Work out the finished part from the listing and answer in its coordinate system (mm). A direction names the side the tool comes from. Give positions to 0.01 mm unless a question says otherwise; leave off trailing zeros. Loops run counter-clockwise (first coordinate to the right, second up) from the corner with the lowest first, then second, coordinate; pieces in that order, holes last. Notation, with made-up numbers: M -9,84 L 7,84 A20 ccw 7,91 Z; hole C 23,85.5 d4. An arc over 180 degrees is marked long. Answer as a JSON object with one key per item and string values. Group by question number.
```python
from build123d import *

# Parameters (mm, degrees)
SKETCH_1_R          = 14
SKETCH_1_R_2        = 1.5
EXTRUDE_1_DEPTH     = 3
SKETCH_2_R          = 5.5
CUT_EXTRUDE_1_DEPTH = 11
CUT_EXTRUDE_2_DEPTH = 11
SKETCH_6_R          = 1.5
CUT_EXTRUDE_3_DEPTH = 11
SKETCH_4_R          = 1.5
EXTRUDE_2_DEPTH     = 3
FILLET_1_R          = 3


with BuildPart() as part:
    # 草图1 → 凸台-拉伸1 (new body)
    # profile 1 of 2: a face of its own
    with BuildSketch(Plane.XY):
        with BuildLine():
            Line((-14, 27.287521581), (-14, 0))
            ThreePointArc((-14, 0), (0, 14), (14, 0))
            Line((14, 0), (14, 27.287521581))
            Line((14, 27.287521581), (-14, 27.287521581))
        make_face()
    # profile 2 of 2: a face of its own
    with BuildSketch(Plane.XY):
        Circle(SKETCH_1_R)
        with Locations((0, -8)):
            Circle(SKETCH_1_R_2, mode=Mode.SUBTRACT)
        with Locations((8, 0)):
            Circle(SKETCH_1_R_2, mode=Mode.SUBTRACT)
        with Locations((-8, 0)):
            Circle(SKETCH_1_R_2, mode=Mode.SUBTRACT)
    extrude(amount=EXTRUDE_1_DEPTH)

    # 草图2 → 切除-拉伸1 (cut)
    with BuildSketch(Plane.XY.offset(3)):
        Circle(SKETCH_2_R)
    extrude(amount=-CUT_EXTRUDE_1_DEPTH, mode=Mode.SUBTRACT)

    # 草图3 → 切除-拉伸2 (cut)
    with BuildSketch(Plane.XY.offset(3)):
        Polygon((14, 27.287521581), (22.040424941, 27.287521581), (22.040424941, 21.507521581), (-23.523215241, 21.507521581), (-23.523215241, 27.287521581), align=None)
    extrude(amount=-CUT_EXTRUDE_2_DEPTH, mode=Mode.SUBTRACT)

    # 草图6 → 切除-拉伸3 (cut)
    with BuildSketch(Plane.XY.offset(3)):
        with Locations((10, 14.007521581)):
            Circle(SKETCH_6_R)
        with Locations((-10, 14.007521581)):
            Circle(SKETCH_6_R)
    extrude(amount=-CUT_EXTRUDE_3_DEPTH, mode=Mode.SUBTRACT)

    # 草图4 → 凸台-拉伸2 (add)
    with BuildSketch(Plane.XY.offset(3)):
        Polygon((14, 21.507521581), (34.450975214, 21.507521581), (34.450975214, 6.507521581), (14, 6.507521581), (-14, 6.507521581), (-34.450975214, 6.507521581), (-34.450975214, 21.507521581), (-14, 21.507521581), align=None)
        with Locations((10, 14.007521581)):
            Circle(SKETCH_4_R, mode=Mode.SUBTRACT)
        with Locations((28, 14.007521581)):
            Circle(SKETCH_4_R, mode=Mode.SUBTRACT)
        with Locations((-10, 14.007521581)):
            Circle(SKETCH_4_R, mode=Mode.SUBTRACT)
        with Locations(Location((-28, 14.007521581, 0), (0, 0, 180))):
            Circle(SKETCH_4_R, mode=Mode.SUBTRACT)
    extrude(amount=-EXTRUDE_2_DEPTH)

    # 圆角1
    fillet_1_edges = [part.edges().sort_by_distance(p)[0] for p in [
        (-34.450975214, 21.507521581, 1.5),
        (-14, 6.507521581, 1.5),
        (34.450975214, 21.507521581, 1.5),
        (14, 6.507521581, 1.5),
        (34.450975214, 6.507521581, 1.5),
        (-34.450975214, 6.507521581, 1.5),
    ]]
    fillet(fillet_1_edges, radius=FILLET_1_R)


solid = part.part
```
Item 1: Find the intervals of material crossed by probe 1 along X at (y, z) = (14, 0.95); probe 2 along Y at (x, z) = (28, 2.3); probe 3 along Y at (x, z) = (8, 1), in increasing order. Write a range as [from, to].
Item 2: A cutting plane is placed at D-D (z = 1.4). Give the number of separate pieces and of enclosed holes in the cut face, and give its area (3 significant figures).
Item 3: Given pin 1 Ø1.5 at (y, z) = (2.5, 2) entering from -X; pin 2 Ø1.5 at (x, z) = (-21, 2) entering from -Y; pin 3 Ø1.5 at (y, z) = (2, 2) entering from +X, each flat-ended and moving along its own axis, determine where each tip first touches the part or whether it passes through.
Item 4: A cutting plane is placed at C-C (y = -8). Determine the outline of the cut face in (x, z).
Item 5: A tool of negligible diameter and unlimited length cuts with its end or side. For faces 4 (the flat face through (-24, 6.508, 2)), 5 (the flat face through (34.451, 14, 2)), 6 (the flat face through (14, 2, 1)), from which of +Z, -Z, +X, -X, +Y, -Y can it reach the whole face along a straight path? Write none if from no direction.
Item 6: A cutting plane is placed at A-A (x = -28). Determine the outline of the cut face in (y, z), and give its area (3 significant figures).
Item 7: For a pull along X with two mould halves and no side action, classify faces 1 (the cylindrical face through (-0.325, -9.464, 1.479)), 2 (the flat face through (0, 12, 0)), 3 (the flat face through (-14, 2, 1)) as pulls with the +X half, pulls with the -X half, needs draft (parallel to the pull), parting line crosses it, or undercut.
Item 8: A cutting plane is placed at B-B (x = 0). Determine the outline of the cut face in (y, z).
The answers:
{
 "1": {"probe 1": "x = [-34.45, -29.5], [-26.5, -11.5], [-8.5, 8.5], [11.5, 26.5], [29.5, 34.45]", "probe 2": "y = [6.51, 12.51], [15.51, 21.51]", "probe 3": "y = [-11.49, -1.5], [1.5, 21.51]"},
 "2": {"separate pieces": "1", "enclosed holes": "8", "area": "1,380 mm^2"},
 "3": {"pin 1": "stops at x = -14", "pin 2": "stops at y = 6.51", "pin 3": "stops at x = 14"},
 "4": {"outline": "M -11.49,0 L -1.5,0 L -1.5,3 L -11.49,3 Z; M 1.5,0 L 11.49,0 L 11.49,3 L 1.5,3 Z"},
 "5": {"face 4": "+Z, -Z, -X, -Y", "face 5": "+Z, -Z, +X, +Y, -Y", "face 6": "+Z, -Z, +X, -Y"},
 "6": {"outline": "M 6.51,0 L 12.51,0 L 12.51,3 L 6.51,3 Z; M 15.51,0 L 21.51,0 L 21.51,3 L 15.51,3 Z", "area": "36.0 mm^2"},
 "7": {"face 1": "undercut", "face 2": "needs draft", "face 3": "pulls with the -X half"},
 "8": {"outline": "M -14,0 L -9.5,0 L -9.5,3 L -14,3 Z; M -6.5,0 L -5.5,0 L -5.5,3 L -6.5,3 Z; M 5.5,0 L 21.51,0 L 21.51,3 L 5.5,3 Z"}
}
